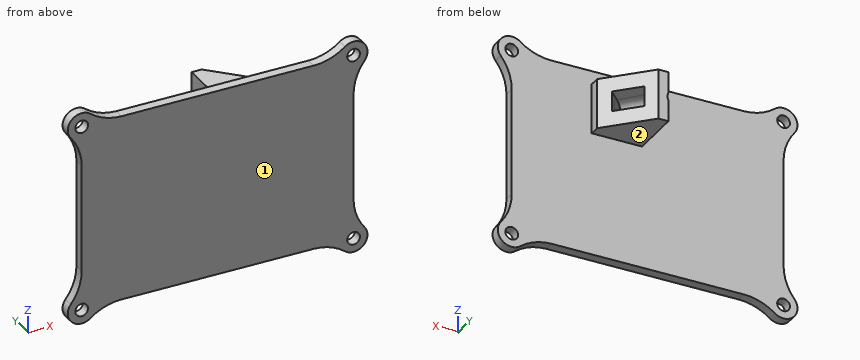
from build123d import *

# Parameters (mm, degrees)
SKETCH1_R           = 4.15
SKETCH1_W           = 81
SKETCH1_H           = 56
BOSS_EXTRUDE1_DEPTH = 3
FILLET1_R           = 15
SKETCH2_R           = 1.9
CUT_EXTRUDE1_DEPTH  = 3
SKETCH3_W           = 15
SKETCH3_H           = 15
BOSS_EXTRUDE2_DEPTH = 15
CHAMFER1_SIZE       = 12
SKETCH4_W           = 6
SKETCH4_H           = 9
CUT_EXTRUDE3_DEPTH  = 5


# Read off the part's stored shape, not the designer's step: Cut-Extrude2
with BuildPart() as part:
    # Sketch1 → Boss-Extrude1 (new body)
    with BuildSketch(Plane(origin=(0, 0, 0), x_dir=(1, 0, 0), z_dir=(0, 1, 0))):
        Circle(SKETCH1_R)
        with Locations((81, 0)):
            Circle(SKETCH1_R)
        with Locations((81, 56)):
            Circle(SKETCH1_R)
        with Locations((0, 56)):
            Circle(SKETCH1_R)
        with Locations((40.5, 28)):
            Rectangle(SKETCH1_W, SKETCH1_H)
        with BuildLine():
            ThreePointArc((76.85, 56), (78.065506858, 53.065506858), (81, 51.85))
            Line((81, 51.85), (81, 56))
            Line((81, 56), (76.85, 56))
        make_face()
        with BuildLine():
            Line((81, 56), (81, 51.85))
            ThreePointArc((81, 51.85), (83.934493142, 53.065506858), (85.15, 56))
            ThreePointArc((85.15, 56), (81, 60.15), (76.85, 56))
            Line((76.85, 56), (81, 56))
        make_face()
        with BuildLine():
            ThreePointArc((81, 4.15), (78.065506858, 2.934493142), (76.85, 0))
            Line((76.85, 0), (81, 0))
            Line((81, 0), (81, 4.15))
        make_face()
        with BuildLine():
            Line((81, 0), (76.85, 0))
            ThreePointArc((76.85, 0), (81, -4.15), (85.15, 0))
            ThreePointArc((85.15, 0), (83.934493142, 2.934493142), (81, 4.15))
            Line((81, 4.15), (81, 0))
        make_face()
        with BuildLine():
            Line((0, 4.15), (0, 0))
            Line((0, 0), (4.15, 0))
            ThreePointArc((4.15, 0), (2.934493142, 2.934493142), (0, 4.15))
        make_face()
        with BuildLine():
            Line((4.15, 0), (0, 0))
            Line((0, 0), (0, 4.15))
            ThreePointArc((0, 4.15), (-2.934493142, -2.934493142), (4.15, 0))
        make_face()
        with BuildLine():
            ThreePointArc((4.15, 56), (-2.934493142, 58.934493142), (0, 51.85))
            Line((0, 51.85), (0, 56))
            Line((0, 56), (4.15, 56))
        make_face()
        with BuildLine():
            Line((0, 56), (0, 51.85))
            ThreePointArc((0, 51.85), (2.934493142, 53.065506858), (4.15, 56))
            Line((4.15, 56), (0, 56))
        make_face()
    extrude(amount=BOSS_EXTRUDE1_DEPTH)

    # Fillet1
    fillet1_edges = [part.edges().sort_by_distance(p)[0] for p in [
        (0, 1.5, -4.15),
        (0, 1.5, -51.85),
        (4.15, 1.5, -56),
        (76.85, 1.5, -56),
        (81, 1.5, -51.85),
        (81, 1.5, -4.15),
        (76.85, 1.5, 0),
        (4.15, 1.5, 0),
    ]]
    fillet(fillet1_edges, radius=FILLET1_R)

    # Sketch2 → Cut-Extrude1 (cut)
    with BuildSketch(Plane(origin=(0, 3, 0), x_dir=(1, 0, 0), z_dir=(0, 1, 0))):
        with Locations(Location((0, 56, 0), (0, 0, 270))):
            Circle(SKETCH2_R)
        with Locations(Location((81, 56, 0), (0, 0, 270))):
            Circle(SKETCH2_R)
        with Locations(Location((81, 0, 0), (0, 0, 270))):
            Circle(SKETCH2_R)
        with Locations(Location((0, 0, 0), (0, 0, 270))):
            Circle(SKETCH2_R)
    extrude(amount=-CUT_EXTRUDE1_DEPTH, mode=Mode.SUBTRACT)

    # Sketch3 → Boss-Extrude2 (add)
    with BuildSketch(Plane(origin=(0, 3, 0), x_dir=(1, 0, 0), z_dir=(0, 1, 0))):
        with Locations((49.654495899, 11.5)):
            Rectangle(SKETCH3_W, SKETCH3_H)
    extrude(amount=BOSS_EXTRUDE2_DEPTH)

    # Chamfer1
    chamfer1_edges = [part.edges().sort_by_distance(p)[0] for p in [
        (57.154495899, 18, -11.5),
    ]]
    chamfer(chamfer1_edges, length=CHAMFER1_SIZE)

    # Cut-Extrude2 outline → Cut-Extrude2 (revolve, cut)
    with BuildSketch(Plane(origin=(27.927971364, 27.927971364, -11.5), x_dir=(0.707106781186549, 0.707106781186546, 0), z_dir=(0, 0, -1))):
        Polygon((3.25, 17.079807846), (3.25, 20.119343944), (3.040539221, 32.119343941), (2e-09, 32.119343946), (0, 17.079807846), align=None)
    revolve(axis=Axis((27.927971364, 27.927971364, -11.5), (0.707106781186546, -0.707106781186549, 0)), mode=Mode.SUBTRACT)

    # Sketch4 → Cut-Extrude3 (cut)
    with BuildSketch(Plane(origin=(31.57724795, 31.57724795, 0), x_dir=(0, 0, -1), z_dir=(0.7071067811865487, 0.7071067811865465, 0))):
        with Locations((11.5, -27.579807846)):
            Rectangle(SKETCH4_W, SKETCH4_H)
    extrude(amount=-CUT_EXTRUDE3_DEPTH, mode=Mode.SUBTRACT)


solid = part.part
Model file for the job. Use its own axes, mm. Face numbers are marked on the shaded views. A direction names the side the tool comes from. Coordinates: 2 decimals unless noted, no trailing zeros. Loops run counter-clockwise (first coordinate to the right, second up) from the corner with the lowest first, then second, coordinate; pieces in that order, holes last. Notation, with made-up numbers: (14, 84) -> (26, 84) arc R28 cw to (26, 108) -> close; hole circle Ø10 at (-32.75, -20.75). An arc over 180 degrees is marked (long way). Use one line per item in the form item = value. Start each with the question number.
(1) Flat gauge pins, fed straight in: pin 1 (4 mm diameter, centred on x = 50, z = -6.5, fed in from +Y); pin 2 (6 mm diameter, centred on x = 0, z = 0, fed in from +Y); pin 3 (5 mm diameter, centred on x = 42, y = 10.5, fed in from -Z). Where does each tip first touch, or does it go through?
(2) Cut at B-B on x = 71.5. Give the cut face in (y, z).
(3) Tool access for the marked faces 1 and 2: list every direction of +Z, -Z, +X, -X, +Y, -Y with a clear straight run to the whole face (end or side of a thin tool).
(4) Probe probe 1 along Z at (x, y) = (50, 9.75); probe 2 along Y at (x, z) = (15, -49.5); probe 3 along Z at (x, y) = (24, 2.75). List the from-to ranges inside material, lowest first. Write a range as from..to.
(5) Cut at A-A on z = -24. Give the cut face in (x, y), and give its area (3 significant figures).
Values:
q1.pin_1 = 15.15
q1.pin_2 = 3
q1.pin_3 = -19
q2.outline = (0, -56.19) -> (3, -56.19) -> (3, 0.19) -> (0, 0.19) -> close
q3.face_1 = +Z, -Z, +X, -X, -Y
q3.face_2 = -Z, +X, -X, +Y
q4.probe_1 = -19..-14.5, -8.5..-4
q4.probe_2 = 0..3
q4.probe_3 = -56..0
q5.outline = (0, 0) -> (81, 0) -> (81, 3) -> (0, 3) -> close
q5.area = 243 mm2
